CAD build for the part. Positions are in the model's coordinates, mm. A direction names the side the tool comes from. Round coordinates to 2 decimals unless told otherwise and drop trailing zeros. Order: outer loops, then holes, each group sorted by start corner. A loop starts at its lowest first (then second) coordinate and runs counter-clockwise, first axis right, second up. Notation, with made-up numbers: (-38.5, 31) - (-7.5, 31) arc R27 cw to (-7.5, 64) - close; hole circle Ø2 at (69.5, 58.5). An arc over 180 degrees is marked (long way). Use one line per item in the form item = value. Start each with the question number.
from build123d import *

# Parameters (mm, degrees)
SKETCH_2_W               = 109.92
SKETCH_2_H               = 76
EXTRUDE_1_DEPTH          = 10
CUT_EXTRUDE_1_DEPTH      = 5
SKETCH_4_R               = 2
CUT_EXTRUDE_2_DEPTH      = 92.808295873
SKETCH_5_W               = 109.92
SKETCH_5_H               = 6
EXTRUDE_2_DEPTH          = 25
CUT_EXTRUDE_3_DEPTH      = 104.340627651
CUT_EXTRUDE_3_DEPTH_BACK = 104.340627651
SKETCH_7_R               = 2.1
SKETCH_9_R               = 2.1
CUT_EXTRUDE_4_DEPTH      = 96.019804204
CUT_EXTRUDE_5_DEPTH      = 5
EXTRUDE_3_DEPTH          = 35
EXTRUDE_4_DEPTH          = 35
SKETCH_13_W              = 46
SKETCH_13_H              = 15
SKETCH_13_W_2            = 12
SKETCH_13_H_2            = 6
CUT_EXTRUDE_6_DEPTH      = 15
CUT_EXTRUDE_7_DEPTH      = 15
SKETCH_15_R              = 1.25
CUT_EXTRUDE_8_DEPTH      = 28.709519
EXTRUDE_5_DEPTH          = 35
CUT_EXTRUDE_10_DEPTH     = 4
CUT_EXTRUDE_11_REACH     = 116.42
SKETCH_22_R              = 2
CUT_EXTRUDE_12_DEPTH     = 3.5
CUT_EXTRUDE_14_REACH     = 117.568
EXTRUDE_6_DEPTH          = 3
FILLET_1_R               = 2


with BuildPart() as part:
    # 草圖2 → 填料-伸長1 (new body)
    with BuildSketch(Plane.XY):
        with Locations((12.52544527, 24.044160626)):
            Rectangle(SKETCH_2_W, SKETCH_2_H)
    extrude(amount=EXTRUDE_1_DEPTH)

    # 草圖3 → 除料-伸長1 (cut)
    with BuildSketch(Plane.XY.offset(10)):
        with BuildLine():
            Line((67.48544527, -6.055839374), (67.48544527, 54.144160626))
            Line((67.48544527, 54.144160626), (61.24181631, 50.538464901))
            ThreePointArc((61.24181631, 50.538464901), (61.408690367, 50.105080914), (61.46544527, 49.644160626))
            ThreePointArc((61.46544527, 49.644160626), (60.088104264, 47.81746208), (57.95299519, 48.639170705))
            Line((57.95299519, 48.639170705), (55.48544527, 47.214160626))
            Line((55.48544527, 47.214160626), (55.48544527, 0.874160626))
            Line((55.48544527, 0.874160626), (57.95299519, -0.550849453))
            ThreePointArc((57.95299519, -0.550849453), (60.088104264, 0.270859171), (61.46544527, -1.555839374))
            ThreePointArc((61.46544527, -1.555839374), (61.408690367, -2.016759663), (61.24181631, -2.45014365))
            Line((61.24181631, -2.45014365), (67.48544527, -6.055839374))
        make_face()
    extrude(amount=-CUT_EXTRUDE_1_DEPTH, mode=Mode.SUBTRACT)

    # 草圖4 → 除料-伸長2 (cut, through all)
    with BuildSketch(Plane.XY.offset(5)):
        with Locations((59.56544527, 41.644160626)):
            Circle(SKETCH_4_R)
        with Locations((59.56544527, 33.644160626)):
            Circle(SKETCH_4_R)
        with Locations((59.56544527, 6.444160626)):
            Circle(SKETCH_4_R)
        with Locations((59.56544527, 14.444160626)):
            Circle(SKETCH_4_R)
    extrude(amount=-CUT_EXTRUDE_2_DEPTH, mode=Mode.SUBTRACT)

    # 草圖5 → 填料-伸長2 (add)
    with BuildSketch(Plane.XY.offset(10)):
        with Locations((12.52544527, -10.955839374)):
            Rectangle(SKETCH_5_W, SKETCH_5_H)
        with Locations((12.52544527, 59.044160626)):
            Rectangle(SKETCH_5_W, SKETCH_5_H)
    extrude(amount=EXTRUDE_2_DEPTH)

    # 草圖7 → 除料-伸長3 (cut, two sides: drawn at the far end of the back side and taken through both)
    with BuildSketch(Plane(origin=(0, -7.955839374, 0), x_dir=(1, 0, 0), z_dir=(0, 1, 0)).offset(-CUT_EXTRUDE_3_DEPTH_BACK)):
        with Locations(Location((-36.43455473, -18, 0), (0, 0, 270))):
            Circle(SKETCH_7_R)
        with Locations(Location((-36.43455473, -26, 0), (0, 0, 270))):
            Circle(SKETCH_7_R)
    extrude(amount=CUT_EXTRUDE_3_DEPTH + CUT_EXTRUDE_3_DEPTH_BACK, mode=Mode.SUBTRACT)

    # 草圖9 → 除料-伸長4 (cut, through all)
    with BuildSketch(Plane.XY.offset(10)):
        with Locations((-36.43455473, 0.044160626)):
            Circle(SKETCH_9_R)
        with Locations((-36.43455473, 8.044160626)):
            Circle(SKETCH_9_R)
        with Locations((-36.43455473, 16.044160626)):
            Circle(SKETCH_9_R)
        with Locations((-36.43455473, 24.044160626)):
            Circle(SKETCH_9_R)
        with Locations((-36.43455473, 32.044160626)):
            Circle(SKETCH_9_R)
        with Locations((-36.43455473, 40.044160626)):
            Circle(SKETCH_9_R)
        with Locations((-36.43455473, 48.044160626)):
            Circle(SKETCH_9_R)
    extrude(amount=-CUT_EXTRUDE_4_DEPTH, mode=Mode.SUBTRACT)

    # 草圖10 → 除料-伸長5 (cut)
    with BuildSketch(Plane(origin=(0, 0, 0), x_dir=(-1, 0, 0), z_dir=(0, 0, -1))):
        with BuildLine():
            Line((32.43455473, 0.044160626), (32.43455473, 48.044160626))
            ThreePointArc((32.43455473, 48.044160626), (36.43455473, 52.044160626), (40.43455473, 48.044160626))
            Line((40.43455473, 48.044160626), (40.43455473, 0.044160626))
            ThreePointArc((40.43455473, 0.044160626), (36.43455473, -3.955839374), (32.43455473, 0.044160626))
        make_face()
    extrude(amount=-CUT_EXTRUDE_5_DEPTH, mode=Mode.SUBTRACT)

    # 草圖11 → 填料-伸長3 (add, through all)
    with BuildSketch(Plane.XY.offset(35)):
        Polygon((51.48544527, 62.044160626), (37.05168854, 87.044160626), (-6.249581649, 62.044160626), align=None)
    extrude(amount=-EXTRUDE_3_DEPTH)

    # 草圖12 → 填料-伸長4 (add)
    with BuildSketch(Plane.XY.offset(35)):
        Polygon((-6.249581649, 62.044160626), (37.05168854, 87.044160626), (47.05168854, 69.72365255), (3.750418351, 44.72365255), align=None)
    extrude(amount=-EXTRUDE_4_DEPTH)

    # 草圖13 → 除料-伸長6 (cut)
    with BuildSketch(Plane(origin=(-28.428305041, 49.239268705, 0), x_dir=(0.8660254037844416, 0.4999999999999949, 0), z_dir=(-0.4999999999999949, 0.8660254037844416, 0))):
        with Locations((50.609783842, -18.9)):
            Rectangle(SKETCH_13_W, SKETCH_13_H)
        with Locations((50.609783842, -29.4)):
            Rectangle(SKETCH_13_W_2, SKETCH_13_H_2)
    extrude(amount=-CUT_EXTRUDE_6_DEPTH, mode=Mode.SUBTRACT)

    # 草圖14 → 除料-伸長7 (cut)
    with BuildSketch(Plane(origin=(0, 0, 32.4), x_dir=(-1, 0, 0), z_dir=(0, 0, -1))):
        Polygon((-22.597205868, 74.080059011), (-27.097205868, 66.285830377), (-16.704901023, 60.285830377), (-12.204901023, 68.080059011), align=None)
    extrude(amount=-CUT_EXTRUDE_7_DEPTH, mode=Mode.SUBTRACT)

    # 草圖15 → 除料-伸長8 (cut)
    with BuildSketch(Plane(origin=(-20.928305041, 36.248887648, 0), x_dir=(0.8660254037844417, 0.4999999999999947, 0), z_dir=(-0.49999999999999484, 0.8660254037844418, 0))):
        with Locations(Location((69.109783842, -18.9, 0), (0, 0, 180))):
            Circle(SKETCH_15_R)
        with Locations(Location((32.109783842, -18.9, 0), (0, 0, 180))):
            Circle(SKETCH_15_R)
    extrude(amount=-CUT_EXTRUDE_8_DEPTH, mode=Mode.SUBTRACT)

    # 草圖18 → 填料-伸長5 (add)
    with BuildSketch(Plane.XY.offset(35)):
        Polygon((-13.593592417, -13.522826672), (-13.343592417, -13.955839374), (-8.724790263, -13.955839374), (-10.129490801, -11.522826672), align=None)
        Polygon((-17.093592417, -7.460648846), (-13.593592417, -13.522826672), (-10.129490801, -11.522826672), (-6.665389186, -9.522826672), (-3.201287571, -7.522826672), (-6.701287571, -1.460648846), align=None)
        Polygon((-3.201287571, -7.522826672), (-6.665389186, -9.522826672), (-4.10598811, -13.955839374), (0.512814044, -13.955839374), align=None)
    extrude(amount=-EXTRUDE_5_DEPTH)

    # 草圖21 → 除料-伸長10 (cut)
    with BuildSketch(Plane(origin=(0, 0, 0), x_dir=(-1, 0, 0), z_dir=(0, 0, -1))):
        Polygon((-37.05168854, 87.044160626), (-43.05168854, 76.65185578), (-51.48544527, 62.044160626), (-17.750418351, 62.044160626), (-11.750418351, 72.436465471), align=None)
    extrude(amount=-CUT_EXTRUDE_10_DEPTH, mode=Mode.SUBTRACT)

    # 草圖22 → 除料-伸長11 (cut, up to next)
    with BuildSketch(Plane(origin=(0, 0, 4), x_dir=(-1, 0, 0), z_dir=(0, 0, -1)), mode=Mode.PRIVATE) as cut_extrude_11_sk1:
        with Locations((-34.12348531, 76.115957396)):
            Circle(SKETCH_22_R)
    cut_extrude_11_tool1 = extrude(cut_extrude_11_sk1.sketch, amount=-CUT_EXTRUDE_11_REACH, mode=Mode.PRIVATE) & part.part
    # 草圖22 → 除料-伸長11 (cut, up to next)
    with BuildSketch(Plane(origin=(0, 0, 4), x_dir=(-1, 0, 0), z_dir=(0, 0, -1)), mode=Mode.PRIVATE) as cut_extrude_11_sk2:
        with Locations((-20.267078849, 68.115957396)):
            Circle(SKETCH_22_R)
    cut_extrude_11_tool2 = extrude(cut_extrude_11_sk2.sketch, amount=-CUT_EXTRUDE_11_REACH, mode=Mode.PRIVATE) & part.part
    add(cut_extrude_11_tool1.solids().sort_by_distance((34.123485, 76.115957, 4))[0], mode=Mode.SUBTRACT)
    add(cut_extrude_11_tool2.solids().sort_by_distance((20.267079, 68.115957, 4))[0], mode=Mode.SUBTRACT)

    # 草圖23 → 除料-伸長12 (cut)
    with BuildSketch(Plane.XY.offset(11.4)):
        Polygon((16.539589727, 69.567103439), (17.14660495, 65.613430145), (20.874094073, 64.162284101), (23.994567972, 66.664811352), (23.387552749, 70.618484646), (19.660063626, 72.06963069), align=None)
        Polygon((30.395996187, 77.567103439), (31.00301141, 73.613430145), (34.730500533, 72.162284101), (37.850974433, 74.664811352), (37.24395921, 78.618484646), (33.516470087, 80.06963069), align=None)
    extrude(amount=-CUT_EXTRUDE_12_DEPTH, mode=Mode.SUBTRACT)

    # 草圖24 → 除料-伸長14 (cut, up to next)
    with BuildSketch(Plane.XY.offset(35), mode=Mode.PRIVATE) as cut_extrude_14_sk1:
        Polygon((-7.570089725, -15.955839374), (-4.10598811, -13.955839374), (-9.165389186, -5.192699653), (-12.629490801, -7.192699653), align=None)
    cut_extrude_14_tool1 = extrude(cut_extrude_14_sk1.sketch, amount=-CUT_EXTRUDE_14_REACH, mode=Mode.PRIVATE) & part.part
    add(cut_extrude_14_tool1.solids().sort_by_distance((-8.367739, -10.57427, 35))[0], mode=Mode.SUBTRACT)

    # 草圖25 → 填料-伸長6 (add)
    with BuildSketch(Plane(origin=(0, 0, 0), x_dir=(-1, 0, 0), z_dir=(0, 0, -1))):
        Polygon((8.724790263, -13.955839374), (4.10598811, -13.955839374), (9.165389186, -5.192699653), (12.629490801, -7.192699653), align=None)
    extrude(amount=-EXTRUDE_6_DEPTH)

    # 圓角1
    fillet_1_edges = [part.edges().sort_by_distance(p)[0] for p in [
        (-24.34206819, 62.044160626, 0),
        (-6.249581649, 62.044160626, 17.5),
        (45.421779388, 56.044160626, 10),
        (0.482469159, 50.383906588, 10),
        (13.554265928, 50.383906588, 10),
        (3.750418351, 44.72365255, 22.5),
        (0.482469159, 50.383906588, 35),
        (13.554265928, 50.383906588, 35),
        (2.750418351, 67.240313048, 0),
        (12.52544527, -13.955839374, 0),
        (32.267078849, -7.955839374, 10),
        (-42.43455473, 24.044160626, 0),
        (-22.610017382, 56.044160626, 10),
        (-42.43455473, 62.044160626, 17.5),
        (-42.43455473, -13.955839374, 17.5),
    ]]
    fillet(fillet_1_edges, radius=FILLET_1_R - 0.0001)  # a hair under: the kernel refuses the full size


solid = part.part
(1) Which spindle directions (+Z, -Z, +X, -X, +Y, -Y) get a long thin tool onto all of the face, cutting with end or side? Do faces 1 (the flat face through (55.485, 24, 8)), 2 (the flat face through (30.7, 75.6, 9.7)), 3 (the cylindrical face through (-36.523, -3.955, 2.465)), 4 (the flat face through (6, 61, 26.4)), 5 (the flat face through (18.98, 64.9, 9.67)). Say none if no direction does.
(2) Mould opens along Z. For faces 6 (the flat face through (12, -10, 35)), 7 (the cylindrical face through (-36.347, 52.043, 2.465)), 8 (the flat face through (32, 75, 26.4)) say: pulls with the +Z half, pulls with the -Z half, needs draft (parallel to the pull), parting line crosses it, or undercut.
(3) Flat gauge pins, fed straight in: P1, Ø1.5, axis at x = -29, y = 33.5, coming from the +Z side; P2, Ø6.5, axis at x = 20.27, y = 68.12, coming from the -Z side; P3, Ø10, axis at x = 27.5, z = 11, coming from the +Y side. Where does each tip first touch, or does it go through?
(4) Slice it at C-C (x = -25). Give the cut face in (y, z).
(5) Wall check: line 1 (Y direction, x = -37, z = 13); line 2 (X direction, y = 60.45, z = 18); line 3 (Z direction, x = 30.5, y = 82). Give the ranges that are in metal, low to high. Write a range as [from, to].
Results list:
q1.face_1 = +Z, +X
q1.face_2 = none
q1.face_3 = -Z
q1.face_4 = +Y
q1.face_5 = +Z
q2.face_6 = pulls with the +Z half
q2.face_7 = needs draft
q2.face_8 = undercut
q3.P1 = 10
q3.P2 = 4
q3.P3 = 84.42
q4.outline = (-13.96, 2) arc R2 ccw to (-11.96, 0) - (60.04, 0) arc R2 ccw to (62.04, 2) - (62.04, 35) - (56.04, 35) - (56.04, 12) arc R2 cw to (54.04, 10) - (-7.96, 10) - (-7.96, 35) - (-13.96, 35) - close
q5.line_1 = [-13.96, -7.96], [56.04, 62.04]
q5.line_2 = [-42.39, -38.53], [-34.33, -3.02], [20.99, 43.9], [45.9, 67.49]
q5.line_3 = [4, 11.4], [26.4, 35]
